Here's how the part is built. I have some questions about the finished solid (model axes, mm). A direction names the side the tool comes from. Round coordinates to 2 decimals unless told otherwise and drop trailing zeros. Write each loop counter-clockwise with the first axis right and the second up, starting at its lowest first coordinate (ties: lowest second). Pieces come first, ordered by that corner, then holes. Notation, with made-up numbers: (25, 44) - (47, 44) arc R25 ccw to (47, 67) - close; hole circle Ø10 at (66, 66.5). An arc over 180 degrees is marked (long way). One line per item, written item: value. Start each with the question number.
Item 1: Imagine slicing it at B-B, the plane z = -23. Please give me the cut outline in (x, y).
Item 2: Thinking about a two-plate mould opening in X: for faces 4 (the face through (128, 0, -54)), 5 (the face through (83.537, 3, -47)), 6 (the face through (89.28, 3.13, -14.49)), 7 (the face through (181.42, 3, -37)), which applies, released by +X, released by -X, zero draft, split by the parting line, or undercut?
Item 3: For faces 1 (the face through (129, 3, -61.998)), 2 (the face through (87, 3, -20.38)), 3 (the face through (164.656, 3, -16)), which set-ups out of +Z, -Z, +X, -X, +Y, -Y let a thin tool reach every point of the face, with its end or its side?
Item 4: Imagine slicing it at D-D, the plane x = 140.5. Please give me the cut outline in (y, z), then the cut area to 3 significant figures.
Item 5: Imagine slicing it at C-C, the plane y = 1.25. Count the separate pieces of the cut face and the enclosed holes in it, then the cut area to 3 significant figures.
Item 6: If I drill on line 1 (Z direction, x = 176, y = 3); line 2 (Z direction, x = 84.5, y = 0.75); line 3 (X direction, y = 4, z = -33.5), over which ranges is the centre line in solid material (lowest first)?
Item 7: For P1, Ø3, axis at x = 80.37, z = -57.93, coming from the -Y side; P2, Ø4, axis at x = 88.79, z = -57.93, coming from the +Y side, each with a flat end and sliding along its axis, tell me the tip position at first contact or that it passes through.
Item 8: Imagine slicing it at A-A, the plane x = 172. Please give me the cut outline in (y, z), then the cut area to 3 significant figures.
```python
from build123d import *

# Parameters (mm, degrees)
SKETCH1_R           = 1.651
BOSS_EXTRUDE1_DEPTH = 6.35
SKETCH2_W           = 12.7
SKETCH2_H           = 3.175
CUT_EXTRUDE7_DEPTH  = 8.89
FILLET2_R           = 1.27
SKETCH4_W           = 3.175
SKETCH4_H           = 19.05
CUT_EXTRUDE8_DEPTH  = 192.82600491
FILLET3_R           = 1.27


with BuildPart() as part:
    # Sketch1 → Boss-Extrude1 (new body)
    with BuildSketch(Plane(origin=(0, 0, 0), x_dir=(1, 0, 0), z_dir=(0, 1, 0))):
        Polygon((75.155177047, 61.997896552), (75.155177047, 11.997896552), (91.919177047, 11.997896552), (91.919177047, 20.379896552), (83.537177047, 20.379896552), (83.537177047, 53.615896552), (173.037829354, 53.615896552), (173.037829354, 20.379896552), (164.655829354, 20.379896552), (164.655829354, 11.997896552), (181.419829354, 11.997896552), (181.419829354, 61.997896552), align=None)
        with Locations(Location((80.3721812, 16.064784874, 0), (0, 0, 270))):
            Circle(SKETCH1_R, mode=Mode.SUBTRACT)
        with Locations(Location((80.3721812, 57.93100823, 0), (0, 0, 270))):
            Circle(SKETCH1_R, mode=Mode.SUBTRACT)
        with Locations(Location((88.7874552, 16.064784874, 0), (0, 0, 270))):
            Circle(SKETCH1_R, mode=Mode.SUBTRACT)
        with Locations(Location((167.7875512, 57.93100823, 0), (0, 0, 270))):
            Circle(SKETCH1_R, mode=Mode.SUBTRACT)
        with Locations(Location((88.7874552, 57.93100823, 0), (0, 0, 270))):
            Circle(SKETCH1_R, mode=Mode.SUBTRACT)
        with Locations(Location((176.2028252, 57.93100823, 0), (0, 0, 270))):
            Circle(SKETCH1_R, mode=Mode.SUBTRACT)
        with Locations(Location((176.2028252, 16.064784874, 0), (0, 0, 270))):
            Circle(SKETCH1_R, mode=Mode.SUBTRACT)
        with Locations(Location((167.7875512, 16.064784874, 0), (0, 0, 270))):
            Circle(SKETCH1_R, mode=Mode.SUBTRACT)
    extrude(amount=BOSS_EXTRUDE1_DEPTH)

    # Sketch2 → Cut-Extrude7 (cut)
    with BuildSketch(Plane(origin=(181.419829354, 0, 0), x_dir=(0, 0, -1), z_dir=(1, 0, 0))):
        with Locations((43.747896552, 4.7625)):
            Rectangle(SKETCH2_W, SKETCH2_H)
    extrude(amount=-CUT_EXTRUDE7_DEPTH, mode=Mode.SUBTRACT)

    # Fillet2
    fillet2_edges = [part.edges().sort_by_distance(p)[0] for p in [
        (177.228829354, 6.35, -37.397896552),
        (177.228829354, 6.35, -50.097896552),
        (177.228829354, 3.175, -50.097896552),
        (177.228829354, 3.175, -37.397896552),
    ]]
    fillet(fillet2_edges, radius=FILLET2_R)

    # Sketch4 → Cut-Extrude8 (cut, through all)
    with BuildSketch(Plane(origin=(0, 6.35, 0), x_dir=(1, 0, 0), z_dir=(0, 1, 0))):
        with Locations((81.949677047, 29.904896552)):
            Rectangle(SKETCH4_W, SKETCH4_H)
    extrude(amount=-CUT_EXTRUDE8_DEPTH, mode=Mode.SUBTRACT)

    # Fillet3
    fillet3_edges = [part.edges().sort_by_distance(p)[0] for p in [
        (83.537177047, 3.175, -39.429896552),
        (80.362177047, 3.175, -20.379896552),
        (80.362177047, 3.175, -39.429896552),
    ]]
    fillet(fillet3_edges, radius=FILLET3_R)


solid = part.part
```
Values follow:
1. outline: (75.16, 0) - (80.36, 0) - (80.36, 6.35) - (75.16, 6.35) - close; (173.04, 0) - (181.42, 0) - (181.42, 6.35) - (173.04, 6.35) - close
2. face 4: zero draft
2. face 5: undercut
2. face 6: undercut
2. face 7: released by +X
3. face 1: -Z, +X, -X, +Y, -Y
3. face 2: +Y, -Y
3. face 3: +Z, +Y, -Y
4. outline: (0, -62) - (6.35, -62) - (6.35, -53.62) - (0, -53.62) - close
4. area: 53.2 mm^2
5. separate pieces: 1
5. enclosed holes: 8
5. area: 1,600 mm^2
6. line 1: z = -62 to -59.57, -56.29 to -17.7, -14.43 to -12
6. line 2: z = -62 to -53.62, -20.38 to -12
6. line 3: x = 75.16 to 80.36, 173.04 to 181.42
7. P1: passes through
7. P2: stops at y = 6.35
8. outline: (0, -62) - (6.35, -62) - (6.35, -53.62) - (0, -53.62) - close; (0, -20.38) - (6.35, -20.38) - (6.35, -12) - (0, -12) - close
8. area: 106 mm^2
